from build123d import *

# Parameters (mm, degrees)
BOSS_EXTRUDE7_DEPTH       = 9
BOSS_EXTRUDE7_DEPTH_BACK  = 50
SKETCH4_R                 = 25
SKETCH4_R_2               = 23
SKETCH20_R                = 8.275
BOSS_EXTRUDE16_DEPTH      = 13
SKETCH24_R                = 2.54
CUT_EXTRUDE10_DEPTH       = 4
SKETCH20_17_R             = 25
BOSS_EXTRUDE17_DEPTH      = 4
CUT_EXTRUDE9_DEPTH        = 30
CUT_EXTRUDE9_DEPTH_BACK   = 30
BOSS_EXTRUDE18_DEPTH      = 20
BOSS_EXTRUDE18_DEPTH_BACK = 15
SKETCH26_R                = 22.95
SKETCH26_R_2              = 21
BOSS_EXTRUDE19_START      = -15
SKETCH27_R                = 25
SKETCH27_R_2              = 21
BOSS_EXTRUDE19_DEPTH      = 15
CHAMFER1_SIZE             = 0.7
CHAMFER1_SIZE2            = 0.490145277
CHAMFER2_SIZE             = 0.7
CHAMFER2_SIZE2            = 0.490145277


with BuildPart() as part:
    # Sketch4 → Boss-Extrude7 (new, two sides: drawn at the far end of the back side and taken through both)
    with BuildSketch(Plane(origin=(0, -5.365491749, 5.365491749), x_dir=(-1, 0, 0), z_dir=(0, 0.7071067811865458, -0.7071067811865492)).offset(-BOSS_EXTRUDE7_DEPTH_BACK)):
        with Locations(Location((0, 0, 0), (0, 0, 90))):
            Circle(SKETCH4_R)
        with Locations(Location((0, 0, 0), (0, 0, 90))):
            Circle(SKETCH4_R_2, mode=Mode.SUBTRACT)
    extrude(amount=BOSS_EXTRUDE7_DEPTH + BOSS_EXTRUDE7_DEPTH_BACK)



with BuildPart() as body_2:
    # Sketch20 → Boss-Extrude16 (new body)
    with BuildSketch(Plane(origin=(0, -40.720830808, 40.720830808), x_dir=(1, 0, 0), z_dir=(0, -0.7071067811865457, 0.7071067811865495))):
        with Locations(Location((0, 0, 0), (0, 0, 270))):
            Circle(SKETCH20_R)
    extrude(amount=BOSS_EXTRUDE16_DEPTH)

    # Sketch24 → Cut-Extrude10 (cut)
    with BuildSketch(Plane(origin=(0, -49.913218964, 49.913218964), x_dir=(1, 0, 0), z_dir=(0, -0.7071067811865457, 0.7071067811865493))):
        with Locations(Location((0, 0, 0), (0, 0, 270))):
            Circle(SKETCH24_R)
    extrude(amount=-CUT_EXTRUDE10_DEPTH, mode=Mode.SUBTRACT)


with BuildPart() as part_1:
    add(part.part)

    add(body_2.part)  # Boss-Extrude17 merges body 2
    # Sketch20<17> → Boss-Extrude17 (add)
    with BuildSketch(Plane(origin=(0, -40.720830808, 40.720830808), x_dir=(1, 0, 0), z_dir=(0, -0.7071067811865457, 0.7071067811865495))):
        with Locations(Location((0, 0, 0), (0, 0, 90))):
            Circle(SKETCH20_17_R)
    extrude(amount=-BOSS_EXTRUDE17_DEPTH)

    # Sketch20<15> → Cut-Extrude9 (cut, two sides: drawn at the far end of the back side and taken through both)
    with BuildSketch(Plane(origin=(0, -40.720830808, 40.720830808), x_dir=(1, 0, 0), z_dir=(0, -0.7071067811865457, 0.7071067811865495)).offset(-CUT_EXTRUDE9_DEPTH_BACK)):
        with BuildLine():
            Line((-2.019900988, 1.54), (2.019900988, 1.54))
            ThreePointArc((2.019900988, 1.54), (2.54, 0), (2.019900988, -1.54))
            Line((2.019900988, -1.54), (-2.019900988, -1.54))
            ThreePointArc((-2.019900988, -1.54), (-2.54, 0), (-2.019900988, 1.54))
        make_face()
    extrude(amount=CUT_EXTRUDE9_DEPTH + CUT_EXTRUDE9_DEPTH_BACK, mode=Mode.SUBTRACT)



with BuildPart() as body_2_2:
    # Sketch26 → Boss-Extrude18 (new, two sides: drawn at the far end of the back side and taken through both)
    with BuildSketch(Plane(origin=(0, 0.998469282, -0.998469282), x_dir=(1, 0, 0), z_dir=(0, 0.7071067811865458, -0.7071067811865492)).offset(-BOSS_EXTRUDE18_DEPTH_BACK)):
        with Locations(Location((0, 0, 0), (0, 0, 270))):
            Circle(SKETCH26_R)
        with Locations(Location((0, 0, 0), (0, 0, 270))):
            Circle(SKETCH26_R_2, mode=Mode.SUBTRACT)
    extrude(amount=BOSS_EXTRUDE18_DEPTH + BOSS_EXTRUDE18_DEPTH_BACK)


with BuildPart() as part_2:
    add(part_1.part)

    add(body_2_2.part)  # Boss-Extrude19 merges body 2 2
    # Sketch27 → Boss-Extrude19 (add)
    with BuildSketch(Plane(origin=(0, 0.998469282, -0.998469282), x_dir=(1, 0, 0), z_dir=(0, 0.7071067811865458, -0.7071067811865492)).offset(BOSS_EXTRUDE19_START)):
        with Locations(Location((0, 0, 0), (0, 0, 270))):
            Circle(SKETCH27_R)
        with Locations(Location((0, 0, 0), (0, 0, 270))):
            Circle(SKETCH27_R_2, mode=Mode.SUBTRACT)
    extrude(amount=BOSS_EXTRUDE19_DEPTH)

    # Chamfer1
    chamfer1_edges = [part_2.edges().sort_by_distance(p)[0] for p in [
        (0, -1.087495723, -31.368705534),
    ]]
    chamfer1_side = [part_2.faces().sort_by_distance(p)[0] for p in [
        (0, -8.158563535, -24.297637722),
    ]]
    chamfer(chamfer1_edges, length=CHAMFER1_SIZE, length2=CHAMFER1_SIZE2, reference=chamfer1_side[0])

    # Chamfer2
    chamfer2_edges = [part_2.edges().sort_by_distance(p)[0] for p in [
        (0, -44.06191035, 55.764527578),
    ]]
    chamfer2_side = [part_2.faces().sort_by_distance(p)[0] for p in [
        (0, -39.465716272, 51.1683335),
    ]]
    chamfer(chamfer2_edges, length=CHAMFER2_SIZE, length2=CHAMFER2_SIZE2, reference=chamfer2_side[0])


solid = part_2.part
Read the model definition and answer for the solid it produces. Units are mm, in the model's axes. A direction names the side the tool comes from. Round coordinates to 2 decimals unless told otherwise and drop trailing zeros.
Q1. Consider probe 1 along Z at (x, y) = (-7, -44.5); probe 2 along Y at (x, z) = (11.5, 49); probe 3 along Z at (x, y) = (19.5, -24). Determine where each line is inside the solid, lowest interval first.
Q2. Each of these flat-tipped pins is pushed along its axis until it touches: pin 1 (6 mm diameter, centred on x = 14, z = 28, fed in from +Y); pin 2 (2 mm diameter, centred on x = -12, y = 19, fed in from +Z); pin 3 (4 mm diameter, centred on y = -5, z = 35.5, fed in from +X); pin 4 (8 mm diameter, centred on x = 2.5, z = -0.5, fed in from +Y). Where does it stop, or does it pass through?
Q3. Determine the mould class of faces 1 (the face through (22.755, 5.614, -9.839)), 2 (the face through (-7.291, 16.629, 14.633)), 3 (the face through (0.028, -43.513, 41.335)) for opening direction X: released by +X, released by -X, zero draft, split by the parting line, or undercut.
Q4. Which of the six approach directions +Z, -Z, +X, -X, +Y, -Y give full straight-line access (tool end or side, diameter ignored) to faces 4 (the face through (-0.028, -41.335, 43.513)), 5 (the face through (-13.2, 26.83, -3.45))?
Output:
1. probe 1: z = 10.56 to 13.52, 31.28 to 36.94, 38.26 to 50.74
1. probe 2: y = -32.44 to -26.78, -20.83 to -17.61
1. probe 3: z = 1.88 to 6.75, 41.25 to 46.12
2. pin 1: stops at y = 5.26
2. pin 2: stops at z = 9.97
2. pin 3: stops at x = 15.56
2. pin 4: stops at y = 31.02
3. face 1: split by the parting line
3. face 2: zero draft
3. face 3: undercut
4. face 4: none
4. face 5: -Z, +X, -X, +Y
